The listing builds one solid part. Answer for the finished solid, in the listing's coordinates (mm). A direction names the side the tool comes from. Round coordinates to 2 decimals unless told otherwise and drop trailing zeros. Order: outer loops, then holes, each group sorted by start corner. A loop starts at its lowest first (then second) coordinate and runs counter-clockwise, first axis right, second up. Notation, with made-up numbers: (76, 22) - (104, 22) arc R31 cw to (104, 53) - close; hole circle Ø3 at (76, 21). An arc over 180 degrees is marked (long way). Use CSV: the item, a comma, the result in double quotes. Start each with the question number.
Item 1: Find section D-D, the plane z = -10.5. Give the vertices of the cut face in (x, y), plus the area to 3 significant figures.
Item 2: Find section A-A, the plane y = 35. Give the vertices of the cut face in (x, z).
Item 3: Find section B-B, the plane x = -65. Give the vertices of the cut face in (y, z), plus the area to 3 significant figures.
Item 4: Determine the mould class of faces 5 (the cylindrical face through (-92.5, 35.1, 1.5)), 6 (the flat face through (1, -30, -15)), 7 (the flat face through (7, -32, 0)) for opening direction Y: +Y half, -Y half, draft (parallel to the pull), parting line (faces both ways), or undercut.
Item 5: For faces 1 (the flat face through (90, 0, -15)), 2 (the flat face through (1, 30, -15)), 3 (the cylindrical face through (87.5, 35.1, 1.5)), 4 (the flat face through (-90, 0, -15)), determine the directions among +Z, -Z, +X, -X, +Y, -Y from which every point of the face is accessible in a straight line to the end or side of a thin tool.
Item 6: Straight lines are drawn through the part: line 1 along Y through (x, z) = (90, 1.1); line 2 along Y through (x, z) = (-58.5, -6); line 3 along Z through (x, y) = (43.5, -31). For each, find the intervals that lie inside material, in ascending order. Write a range as [from, to].
Item 7: Flat-ended cylindrical pins translate along their axes: P1, Ø4.5, axis at x = 90, y = -35, coming from the +Z side; P2, Ø10, axis at x = -76, z = -21.5, coming from the +Y side; P3, Ø8, axis at x = 13, z = -18, coming from the -Y side; P4, Ø2, axis at y = 15, z = -10.5, coming from the +X side. Find the tip coordinate at first contact, or state that the pin passes through.
Item 8: Find section C-C, the plane y = -8.5. Give the vertices of the cut face in (x, z).
```python
from build123d import *

# Parameters (mm, degrees)
SKETCH_1_W             = 200
SKETCH_1_H             = 80
EXTRUDE_1_DEPTH        = 3
SKETCH_2_W             = 180
SKETCH_2_H             = 60
EXTRUDE_2_DEPTH        = 30
HOLE_WIZARD_M6_1_D     = 5
HOLE_WIZARD_M6_1_DEPTH = 15
HOLE_WIZARD_M6_1_TIP   = 1.502151548


with BuildPart() as part:
    # 草图1 → 凸台-拉伸1 (new body)
    with BuildSketch(Plane.XY):
        Rectangle(SKETCH_1_W, SKETCH_1_H)
    extrude(amount=EXTRUDE_1_DEPTH)

    # 草图2 → 凸台-拉伸2 (add)
    with BuildSketch(Plane(origin=(0, 0, 0), x_dir=(-1, 0, 0), z_dir=(0, 0, -1))):
        Rectangle(SKETCH_2_W, SKETCH_2_H)
    extrude(amount=EXTRUDE_2_DEPTH)

    # M6 螺纹孔1
    with Locations(Plane(origin=(0, 0, 0), x_dir=(-1, 0, 0), z_dir=(0, 0, -1))):
        with Locations((-90, 35), (-90, -35), (90, -35), (90, 35)):
            Hole(HOLE_WIZARD_M6_1_D / 2, depth=HOLE_WIZARD_M6_1_DEPTH)
            with Locations((0, 0, -(HOLE_WIZARD_M6_1_DEPTH + HOLE_WIZARD_M6_1_TIP / 2))):  # 118° drill point
                Cone(0, HOLE_WIZARD_M6_1_D / 2, HOLE_WIZARD_M6_1_TIP, mode=Mode.SUBTRACT)


solid = part.part
```
Worked out:
1,outline,"(-90, -30) - (90, -30) - (90, 30) - (-90, 30) - close"
1,area,"10,800 mm²"
2,outline,"(-100, 0) - (-92.5, 0) - (-92.5, 3) - (-100, 3) - close; (-87.5, 0) - (87.5, 0) - (87.5, 3) - (-87.5, 3) - close; (92.5, 0) - (100, 0) - (100, 3) - (92.5, 3) - close"
3,outline,"(-40, 0) - (-30, 0) - (-30, -30) - (30, -30) - (30, 0) - (40, 0) - (40, 3) - (-40, 3) - close"
3,area,"2,040 mm²"
4,face 5,"undercut"
4,face 6,"-Y half"
4,face 7,"draft"
5,face 1,"-Z, +X, +Y, -Y"
5,face 2,"-Z, +X, -X, +Y"
5,face 3,"+Z, -Z"
5,face 4,"-Z, -X, +Y, -Y"
6,line 1,"y = [-40, -37.5], [-32.5, 32.5], [37.5, 40]"
6,line 2,"y = [-30, 30]"
6,line 3,"z = [0, 3]"
7,P1,"passes through"
7,P2,"stops at y = 30"
7,P3,"stops at y = -30"
7,P4,"stops at x = 90"
8,outline,"(-100, 0) - (-90, 0) - (-90, -30) - (90, -30) - (90, 0) - (100, 0) - (100, 3) - (-100, 3) - close"
